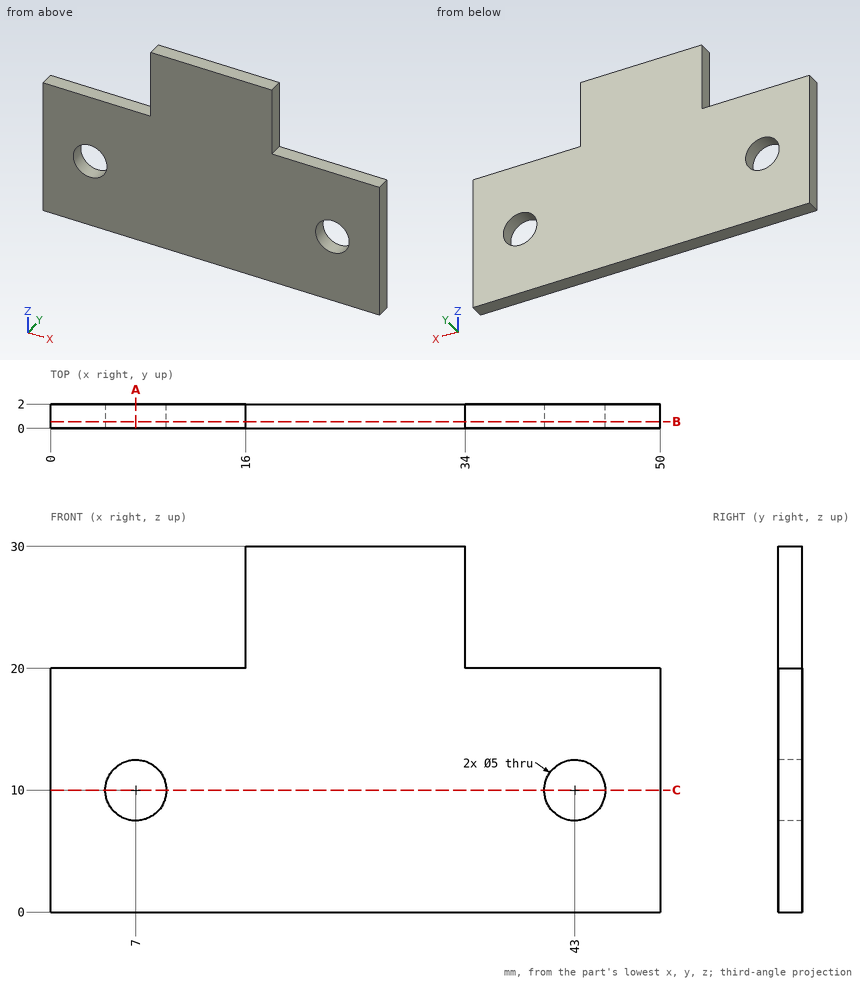
Answer from the drawing. Dimensions are ordinates in mm from the lowest x, y and z of the part. Round coordinates to 2 decimals unless told otherwise and drop trailing zeros. Write each loop counter-clockwise with the first axis right and the second up, starting at its lowest first coordinate (ties: lowest second). Pieces come first, ordered by that corner, then holes. Notation, with made-up numbers: (18.5, 57) -> (72.5, 57) arc R13 cw to (72.5, 69) -> close; hole circle Ø4 at (58.25, 34). An arc over 180 degrees is marked (long way). Write each question's results on one line, items separated by ' | '.
1) The part is cut by section A-A (x = 7). Write down the section's boundary in (y, z), and give its area (3 significant figures).
Findings:
outline: (0, 0) -> (2, 0) -> (2, 7.5) -> (0, 7.5) -> close; (0, 12.5) -> (2, 12.5) -> (2, 20) -> (0, 20) -> close | area: 30.0 mm²
2) Consider line 1 along X through (y, z) = (1.1, 10); line 2 along Z through (x, y) = (7, 1.3); line 3 along Z through (x, y) = (10.5, 0.6). Determine where each line is inside the solid, lowest interval first. Write a range as [from, to].
Findings:
line 1: x = [0, 4.5], [9.5, 40.5], [45.5, 50] | line 2: z = [0, 7.5], [12.5, 20] | line 3: z = [0, 20]
3) Flat-ended cylindrical pins translate along their axes: pin 1 (0.6 mm diameter, centred on x = 41, y = 0.5, fed in from +Z); pin 2 (0.6 mm diameter, centred on y = 1, z = 23.5, fed in from +X). Find the tip coordinate at first contact, or state that the pin passes through.
Findings:
pin 1: stops at z = 20 | pin 2: stops at x = 34
4) The part is cut by section B-B (y = 0.55). Write down the section's boundary in (x, z), and give its area (3 significant figures).
Findings:
outline: (0, 0) -> (50, 0) -> (50, 20) -> (34, 20) -> (34, 30) -> (16, 30) -> (16, 20) -> (0, 20) -> close; hole circle Ø5 at (7, 10); hole circle Ø5 at (43, 10) | area: 1,140 mm²
5) The part is cut by section C-C (z = 10). Write down the section's boundary in (x, y).
Findings:
outline: (0, 0) -> (4.5, 0) -> (4.5, 2) -> (0, 2) -> close; (9.5, 0) -> (40.5, 0) -> (40.5, 2) -> (9.5, 2) -> close; (45.5, 0) -> (50, 0) -> (50, 2) -> (45.5, 2) -> close
